Can you work these out from the model? Positions are in its coordinate system, mm. A direction names the side the tool comes from. Coordinates: 2 decimals unless noted, no trailing zeros. Loops run counter-clockwise (first coordinate to the right, second up) from the corner with the lowest first, then second, coordinate; pieces in that order, holes last. Notation, with made-up numbers: (-7, 84.5) -> (12, 84.5) arc R19 cw to (12, 88.5) -> close; hole circle Ø4 at (-31.75, 29.5). An arc over 180 degrees is marked (long way). Put each result on its own line as item: value. Start each with the question number.
Item 1: Please list where these lines run through material, in increasing order: L1, parallel to Z at x = -1, y = 27.5; L2, parallel to Y at x = 75, z = 12.5. Write a range as from..to.
Item 2: If we section it at B-B on x = 128.5: Please give me the cut outline in (y, z).
Item 3: Will these pins go through, and if not, where does the flat tip stop? P1, Ø2, axis at x = 55, z = 18.5, coming from the -Y side; P2, Ø5, axis at x = 17, y = 13.5, coming from the -Z side; P3, Ø12, axis at x = 106.5, z = -15, coming from the +Y side.
Item 4: If we section it at C-C on y = 32.5: Please give me the cut outline in (x, z).
Item 5: For faces 4 (the cylindrical face through (-4.14, 21.92, 18.99)), 5 (the flat face through (38, 2, -1)), 6 (the flat face through (155, 12, 19)), 7 (the cylindrical face through (-4.13, 0.99, 0.09)), which set-ups out of +Z, -Z, +X, -X, +Y, -Y let a thin tool reach every point of the face, with its end or its side?
Item 6: We'd pull the mould along Z, two halves only. Please class faces 1 (the cylindrical face through (46.65, 22.1, 18.99)), 2 (the flat face through (38, 21, 20)), 3 (the cylindrical face through (-69.32, 0.99, -0.09)): pulls with the +Z half, pulls with the -Z half, needs draft (parallel to the pull), parting line crosses it, or undercut.
Item 7: If we section it at A-A on z = 0: Please give me the cut outline in (x, y).
```python
from build123d import *

# Parameters (mm, degrees)
SKETCH1_W           = 150
SKETCH1_H           = 40
BOSS_EXTRUDE1_DEPTH = 2
SKETCH2_W           = 150
SKETCH2_H           = 2
BOSS_EXTRUDE2_DEPTH = 40
BOSS_EXTRUDE3_DEPTH = 80
CUT_EXTRUDE1_DEPTH  = 10
CUT_EXTRUDE2_DEPTH  = 10


with BuildPart() as part:
    # Sketch1 → Boss-Extrude1 (new body)
    with BuildSketch(Plane(origin=(0, 0, 0), x_dir=(1, 0, 0), z_dir=(0, 1, 0))):
        Rectangle(SKETCH1_W, SKETCH1_H)
    extrude(amount=BOSS_EXTRUDE1_DEPTH)

    # Sketch2 → Boss-Extrude2 (add)
    with BuildSketch(Plane(origin=(0, 2, 0), x_dir=(1, 0, 0), z_dir=(0, 1, 0))):
        with Locations((0, -19)):
            Rectangle(SKETCH2_W, SKETCH2_H)
    extrude(amount=BOSS_EXTRUDE2_DEPTH)

    # Sketch5 → Boss-Extrude3 (add)
    with BuildSketch(Plane(origin=(75, 0, 0), x_dir=(0, 0, -1), z_dir=(1, 0, 0))):
        Polygon((-20, 0), (20, 0), (20, 2), (-18, 2), (-18, 42), (-20, 42), align=None)
    extrude(amount=BOSS_EXTRUDE3_DEPTH)

    # Sketch6 → Cut-Extrude1 (cut)
    with BuildSketch(Plane(origin=(0, 0, 18), x_dir=(-1, 0, 0), z_dir=(0, 0, -1))):
        with BuildLine():
            Line((-105.923719426, 25.947585899), (-88.587761645, 25.947585899))
            ThreePointArc((-88.587761645, 25.947585899), (-84.649216654, 22.009040908), (-88.587761645, 18.070495916))
            Line((-88.587761645, 18.070495916), (-105.923719426, 18.070495916))
            ThreePointArc((-105.923719426, 18.070495916), (-109.862264418, 22.009040908), (-105.923719426, 25.947585899))
        make_face()
        with BuildLine():
            Line((-143.923719426, 25.947585899), (-126.587761645, 25.947585899))
            ThreePointArc((-126.587761645, 25.947585899), (-122.649216654, 22.009040908), (-126.587761645, 18.070495916))
            Line((-126.587761645, 18.070495916), (-143.923719426, 18.070495916))
            ThreePointArc((-143.923719426, 18.070495916), (-147.862264418, 22.009040908), (-143.923719426, 25.947585899))
        make_face()
        with BuildLine():
            Line((-67.923719426, 25.947585899), (-50.587761645, 25.947585899))
            ThreePointArc((-50.587761645, 25.947585899), (-46.649216654, 22.009040908), (-50.587761645, 18.070495916))
            Line((-50.587761645, 18.070495916), (-67.923719426, 18.070495916))
            ThreePointArc((-67.923719426, 18.070495916), (-71.862264418, 22.009040908), (-67.923719426, 25.947585899))
        make_face()
        with BuildLine():
            Line((-29.923719426, 25.947585899), (-12.587761645, 25.947585899))
            ThreePointArc((-12.587761645, 25.947585899), (-8.649216654, 22.009040908), (-12.587761645, 18.070495916))
            Line((-12.587761645, 18.070495916), (-29.923719426, 18.070495916))
            ThreePointArc((-29.923719426, 18.070495916), (-33.862264418, 22.009040908), (-29.923719426, 25.947585899))
        make_face()
        with BuildLine():
            Line((8.076280574, 25.947585899), (25.412238355, 25.947585899))
            ThreePointArc((25.412238355, 25.947585899), (29.350783346, 22.009040908), (25.412238355, 18.070495916))
            Line((25.412238355, 18.070495916), (8.076280574, 18.070495916))
            ThreePointArc((8.076280574, 18.070495916), (4.137735582, 22.009040908), (8.076280574, 25.947585899))
        make_face()
        with BuildLine():
            Line((46.076280574, 25.947585899), (63.412238355, 25.947585899))
            ThreePointArc((63.412238355, 25.947585899), (67.350783346, 22.009040908), (63.412238355, 18.070495916))
            Line((63.412238355, 18.070495916), (46.076280574, 18.070495916))
            ThreePointArc((46.076280574, 18.070495916), (42.137735582, 22.009040908), (46.076280574, 25.947585899))
        make_face()
    extrude(amount=-CUT_EXTRUDE1_DEPTH, mode=Mode.SUBTRACT)

    # Sketch7 → Cut-Extrude2 (cut)
    with BuildSketch(Plane.XZ):
        with BuildLine():
            Line((-27.006843458, 4.316067859), (-8.446451171, 4.316067859))
            ThreePointArc((-8.446451171, 4.316067859), (-4.130383312, 0), (-8.446451171, -4.316067859))
            Line((-8.446451171, -4.316067859), (-27.006843458, -4.316067859))
            ThreePointArc((-27.006843458, -4.316067859), (-31.322911318, 0), (-27.006843458, 4.316067859))
        make_face()
        with BuildLine():
            Line((-65.006843458, 4.316067859), (-46.446451171, 4.316067859))
            ThreePointArc((-46.446451171, 4.316067859), (-42.130383312, 0), (-46.446451171, -4.316067859))
            Line((-46.446451171, -4.316067859), (-65.006843458, -4.316067859))
            ThreePointArc((-65.006843458, -4.316067859), (-69.322911318, 0), (-65.006843458, 4.316067859))
        make_face()
        with BuildLine():
            Line((10.993156542, 4.316067859), (29.553548829, 4.316067859))
            ThreePointArc((29.553548829, 4.316067859), (33.869616688, 0), (29.553548829, -4.316067859))
            Line((29.553548829, -4.316067859), (10.993156542, -4.316067859))
            ThreePointArc((10.993156542, -4.316067859), (6.677088682, 0), (10.993156542, 4.316067859))
        make_face()
        with BuildLine():
            Line((48.993156542, 4.316067859), (67.553548829, 4.316067859))
            ThreePointArc((67.553548829, 4.316067859), (71.869616688, 0), (67.553548829, -4.316067859))
            Line((67.553548829, -4.316067859), (48.993156542, -4.316067859))
            ThreePointArc((48.993156542, -4.316067859), (44.677088682, 0), (48.993156542, 4.316067859))
        make_face()
        with BuildLine():
            Line((86.993156542, 4.316067859), (105.553548829, 4.316067859))
            ThreePointArc((105.553548829, 4.316067859), (109.869616688, 0), (105.553548829, -4.316067859))
            Line((105.553548829, -4.316067859), (86.993156542, -4.316067859))
            ThreePointArc((86.993156542, -4.316067859), (82.677088682, 0), (86.993156542, 4.316067859))
        make_face()
        with BuildLine():
            Line((124.993156542, 4.316067859), (143.553548829, 4.316067859))
            ThreePointArc((143.553548829, 4.316067859), (147.869616688, 0), (143.553548829, -4.316067859))
            Line((143.553548829, -4.316067859), (124.993156542, -4.316067859))
            ThreePointArc((124.993156542, -4.316067859), (120.677088682, 0), (124.993156542, 4.316067859))
        make_face()
    extrude(amount=-CUT_EXTRUDE2_DEPTH, mode=Mode.SUBTRACT)


solid = part.part
```
Solutions:
1. L1: 18..20
1. L2: 0..2
2. outline: (0, -20) -> (2, -20) -> (2, -4.32) -> (0, -4.32) -> close; (0, 4.32) -> (2, 4.32) -> (2, 18) -> (18.07, 18) -> (18.07, 20) -> (0, 20) -> close; (25.95, 18) -> (42, 18) -> (42, 20) -> (25.95, 20) -> close
3. P1: y = 0
3. P2: z = 18
3. P3: y = 2
4. outline: (-75, 18) -> (155, 18) -> (155, 20) -> (-75, 20) -> close
5. face 4: +Z, -Z
5. face 5: -Z, +X, -X, +Y
5. face 6: +Z, -Z, +X, +Y, -Y
5. face 7: +Y, -Y
6. face 1: needs draft
6. face 2: pulls with the +Z half
6. face 3: undercut
7. outline: (-75, 0) -> (-69.32, 0) -> (-69.32, 2) -> (-75, 2) -> close; (-42.13, 0) -> (-31.32, 0) -> (-31.32, 2) -> (-42.13, 2) -> close; (-4.13, 0) -> (6.68, 0) -> (6.68, 2) -> (-4.13, 2) -> close; (33.87, 0) -> (44.68, 0) -> (44.68, 2) -> (33.87, 2) -> close; (71.87, 0) -> (82.68, 0) -> (82.68, 2) -> (71.87, 2) -> close; (109.87, 0) -> (120.68, 0) -> (120.68, 2) -> (109.87, 2) -> close; (147.87, 0) -> (155, 0) -> (155, 2) -> (147.87, 2) -> close
